```python
from build123d import *

# Parameters (mm, degrees)
F0_W     = 30
F0_H     = 30
F1_DEPTH = 4
F2_R     = 3
F3_R     = 7
F4_DEPTH = 14
F5_SIZE  = 2
F6_SIZE  = 1


with BuildPart() as f1:
    # F0 (on Top) → F1 (new body)
    with BuildSketch(Plane.XY):
        Rectangle(F0_W, F0_H)
    extrude(amount=F1_DEPTH)

    # F2
    f2_edges = [f1.edges().sort_by_distance(p)[0] for p in [
        (15, 15, 2),
        (-15, 15, 2),
        (-15, -15, 2),
        (15, -15, 2),
    ]]
    fillet(f2_edges, radius=F2_R)

    # F3 (on face) → F4 (join)
    with BuildSketch(Plane.XY.offset(4)):
        Circle(F3_R)
    extrude(amount=F4_DEPTH)

    # F5
    f5_edges = [f1.edges().sort_by_distance(p)[0] for p in [
        (-7, 0, 18),
        (-7, 0, 4),
    ]]
    chamfer(f5_edges, length=F5_SIZE)

    # F6
    f6_edges = [f1.edges().sort_by_distance(p)[0] for p in [
        (0, -15, 4),
    ]]
    chamfer(f6_edges, length=F6_SIZE)


solid = f1.part
```
Input: part model. Units: mm. Frame: model coordinates. A direction names the side the tool comes from. Give positions to 0.01 mm unless a question says otherwise; leave off trailing zeros. Order: outer loops, then holes, each group sorted by start corner. A loop starts at its lowest first (then second) coordinate and runs counter-clockwise, first axis right, second up. Notation, with made-up numbers: M 66,31 L 99,31 A27 cw 99,59 Z; hole C -39.75,88 d2. An arc over 180 degrees is marked long. One line per question, with ' | ' between items. Start each with the question number.
1. Section query C-C (z = 5.5). Return the cut outline in (x, y).
2. Section query A-A (y = 0). Return the cut outline in (x, z), and give its area (3 significant figures).
3. Access query for faces 1 (the face through (0, 10, 4)), 2 (the face through (-15, 0, 1)). Directions: +Z, -Z, +X, -X, +Y, -Y. A direction counts if a zero-diameter tool reaches every point of the face in a straight line with its end or side. Return the directions, or none.
4. First-contact query: pin 1 Ø1 at (x, y) = (-10, 2) entering from +Z; pin 2 Ø2 at (y, z) = (2.5, 14) entering from -X; pin 3 Ø10 at (x, y) = (-2, 10.5) entering from +Z. Flat tips, straight axial feed; report the tip coordinate or a pass-through.
5. Section query D-D (z = 15). Return the cut outline in (x, y).
6. Material intervals for probe 1 along Z at (x, y) = (-8.5, -8); probe 2 along Y at (x, z) = (4, 16.5); probe 3 along Y at (x, z) = (-2.75, 14.5), sorted ascending. Write a range as [from, to].
Here are the results:
1) outline: C 0,0 d15
2) outline: M -15,0 L 15,0 L 15,3 L 14,4 L 9,4 L 7,6 L 7,16 L 5,18 L -5,18 L -7,16 L -7,6 L -9,4 L -14,4 L -15,3 Z | area: 315 mm²
3) face 1: +Z | face 2: +Z, -Z, -X, +Y, -Y
4) pin 1: z = 4 | pin 2: x = -6.84 | pin 3: z = 17.31
5) outline: C 0,0 d14
6) probe 1: [0, 4] | probe 2: [-5.12, 5.12] | probe 3: [-6.44, 6.44]
